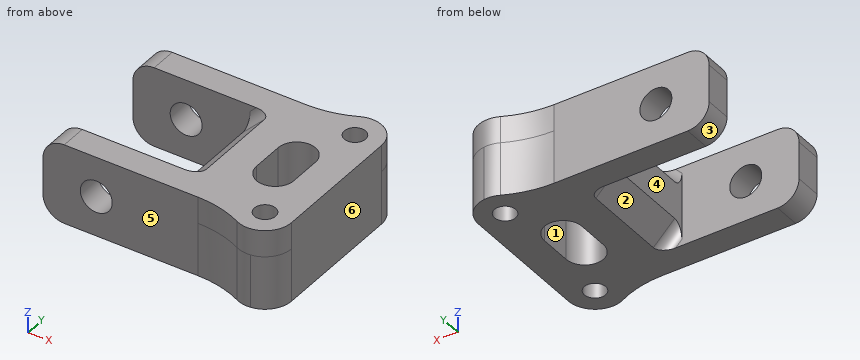
Autodesk Inventor part; units mm, degrees
ref_plane "YZ Plane" through (0, 0, 0) normal (1, 0, 0) x (0, 1, 0)
ref_plane "XZ Plane" through (0, 0, 0) normal (0, 1, 0) x (-1, 0, 0)
ref_plane "XY Plane" through (0, 0, 0) normal (0, 0, 1) x (1, 0, 0)
sketch "Sketch1" plane through (0, 0, 0) normal (0, 0, 1) x (1, 0, 0)
  circle A0 centre (19.8085, -5.5) radius 1
  circle A1 centre (30.8085, -5.5) radius 1
  circle A2 centre (19.8085, 5.5) radius 1
  circle A3 centre (30.8085, 5.5) radius 1
  circle A4 centre (25.3085, 0) radius 6.65
  line L0 (41.3085, 2) -> (41.3085, -2)
  line L1 (35.1065, 2) -> (41.3085, 2)
  arc A5 (35.1065, 2) -> (26.5426, 9.9236) centre (25.3085, 0) ccw
  line L2 (26.5426, 9.9236) -> (-34.0744, 17.4618)
  arc A6 (-34.0744, 17.4618) -> (-39.6915, 12.5) centre (-34.6915, 12.5) ccw
  line L3 (-39.6915, 12.5) -> (-39.6915, -12.5)
  arc A7 (-39.6915, -12.5) -> (-34.0744, -17.4618) centre (-34.6915, -12.5) ccw
  line L4 (-34.0744, -17.4618) -> (26.5426, -9.9236)
  arc A8 (26.5426, -9.9236) -> (35.1065, -2) centre (25.3085, 0) ccw
  line L5 (41.3085, -2) -> (35.1065, -2)
  circle A9 centre (-34.6915, 12.5) radius 2
  circle A10 centre (-34.6915, -12.5) radius 2
  line L6 (-25.1979, 6.2809) -> (9.3489, 1.9847)
  arc A11 (9.3489, -1.9847) -> (9.3489, 1.9847) centre (9.1021, 0) ccw
  line L7 (9.3489, -1.9847) -> (-25.1979, -6.2809)
  arc A12 (-29.6915, -2.3115) -> (-25.1979, -6.2809) centre (-25.6915, -2.3115) ccw
  line L8 (-29.6915, -2.3115) -> (-29.6915, 2.3115)
  arc A13 (-25.1979, 6.2809) -> (-29.6915, 2.3115) centre (-25.6915, 2.3115) ccw
  circle A14 centre (-34.6915, -12.5) radius 5
  circle A15 centre (-34.6915, 12.5) radius 5
  line L9 (-34.6915, -12.5) -> (-34.6915, 12.5)
  line L10 (-34.6915, -12.5) -> (-29.6915, -12.5)
  line L11 (-34.6915, 12.5) -> (-29.6915, 12.5)
  line L12 (-29.6915, 12.5) -> (-29.6915, -12.5)
  line L13 (-34.6915, 0) -> (-64.6915, 0)
  line L14 (-64.6915, -10) -> (-64.6915, 10)
  line L15 (-64.6915, 10) -> (-34.6915, 10)
  line L16 (-34.6915, 10) -> (-34.6915, -10)
  line L17 (-34.6915, -10) -> (-64.6915, -10)
  line L18 (-64.6915, -10) -> (-34.6915, 10) construction
  line L19 (-64.6915, 10) -> (-34.6915, -10) construction
  line L20 (-64.6915, -10) -> (-34.6915, -10)
  line L21 (-34.6915, -10) -> (-34.6915, -15)
  line L22 (-34.6915, -15) -> (-64.6915, -15)
  line L23 (-64.6915, -15) -> (-64.6915, -10)
  line L24 (-64.6915, 10) -> (-34.6915, 10)
  line L25 (-34.6915, 10) -> (-34.6915, 15)
  line L26 (-34.6915, 15) -> (-64.6915, 15)
  line L27 (-64.6915, 15) -> (-64.6915, 10)
  point P0 (0, 0)
  point P1 (-49.6915, 0)
  point P2 (-39.0216, 15)
  point P3 (-39.6915, 10)
  point P4 (-39.6915, -10)
  point P5 (-39.0216, -15)
  dimension "d0" = 10
  dimension "d1" = 10
  dimension "d2" = 30
  dimension "d3" = 20
  dimension "d4" = 30
  dimension "d5" = 30
  dimension "d6" = 5
  dimension "d7" = 30
  dimension "d8" = 5
extrude "Extrusion1" add sketch "Sketch1" along normal blind 10 contours A15 L11 A9 L25 L26 A6 | A7 L22 L21 A10 L10 A14 | L26 L25 A9 L9 L15 A15 A6 | A6 L3 L15 L27 L26 | L12 L8 A14 L9 A15 | A15 L9 A9 L11 | L22 L23 L17 L3 A7 | A7 A14 L17 L9 A10 L21 L22 | L10 A10 L9 A14 | A15 L15 L3 | L9 L13 L3 L15 A15 | A15 L15 L9 | L3 L17 A14 | L9 L17 A14 | A14 L17 L3 L13 L9
thicken "Thicken1" operation add thickness 10 both sides no extend neighbours yes toward (-1, 0, 0) faces at (-64.6915, -11.6667, 3.3333)
thicken "Thicken2" operation add thickness 10 both sides no extend neighbours yes toward (-1, 0, 0) faces at (-64.6915, 13.3333, 3.3333)
sketch "Sketch2" plane through (0, 0, 10) normal (0, 0, 1) x (1, 0, 0)
  line L0 (-39.6915, 10) -> (-39.6915, -10)
  line L1 (-39.6915, -10) -> (-74.6915, -10)
  line L2 (-74.6915, -10) -> (-74.6915, -15)
  line L3 (-74.6915, -15) -> (-39.0216, -15)
  arc A0 (-39.0216, -15) -> (-29.6915, -12.5) centre (-34.6915, -12.5) ccw
  line L4 (-29.6915, -12.5) -> (-29.6915, 12.5)
  arc A1 (-29.6915, 12.5) -> (-39.0216, 15) centre (-34.6915, 12.5) ccw
  line L5 (-39.0216, 15) -> (-74.6915, 15)
  line L6 (-74.6915, 15) -> (-74.6915, 10)
  line L7 (-74.6915, 10) -> (-39.6915, 10)
  circle A2 centre (-34.6915, -12.5) radius 2
  circle A3 centre (-34.6915, 12.5) radius 2
  point P0 (0, 0)
extrude "Extrusion2" add sketch "Sketch2" along normal blind 5
sketch "Sketch3" plane through (0, 0, 15) normal (0, 0, 1) x (1, 0, 0)
  line L0 (-39.6915, 10) -> (-39.6915, -10)
  line L1 (-39.6915, -10) -> (-74.6915, -10)
  line L2 (-74.6915, -10) -> (-74.6915, -15)
  line L3 (-74.6915, -15) -> (-39.0216, -15)
  arc A0 (-39.0216, -15) -> (-29.6915, -12.5) centre (-34.6915, -12.5) ccw
  line L4 (-29.6915, -12.5) -> (-29.6915, 12.5)
  arc A1 (-29.6915, 12.5) -> (-39.0216, 15) centre (-34.6915, 12.5) ccw
  line L5 (-39.0216, 15) -> (-74.6915, 15)
  line L6 (-74.6915, 15) -> (-74.6915, 10)
  line L7 (-74.6915, 10) -> (-39.6915, 10)
  circle A2 centre (-34.6915, -12.5) radius 2
  circle A3 centre (-34.6915, 12.5) radius 2
  line L8 (-39.6915, 10) -> (-39.6915, -10)
  line L9 (-39.6915, 10) -> (-52.6915, 10)
  line L10 (-52.6915, 10) -> (-52.6915, -10)
  line L11 (-52.6915, -10) -> (-39.6915, -10)
  line L12 (-39.6915, -10) -> (-39.6915, 10)
  point P0 (0, 0)
  dimension "d17" = 13
  dimension "d18" = 20
extrude "Extrusion3" add sketch "Sketch3" against normal up to surface (15 mm away) contours L0 L1 L10 L7
chamfer "Chamfer1" distance 4 angle 45 2 edges at (-52.6915, 0, 0) (-52.6915, 0, 15)
fillet "Fillet1" radius 20 2 edges at (-39.0216, -15, 7.5) (-39.0216, 15, 7.5)
sketch "Sketch4" plane through (0, 0, 15) normal (0, 0, 1) x (1, 0, 0)
  line L0 (-48.6915, -10) -> (-74.6915, -10)
  line L1 (-74.6915, -10) -> (-74.6915, -15)
  line L2 (-74.6915, -15) -> (-45.5887, -15)
  arc A0 (-36.8709, -17) -> (-45.5887, -15) centre (-45.5887, -35) ccw
  arc A1 (-36.8709, -17) -> (-29.6915, -12.5) centre (-34.6915, -12.5) ccw
  line L3 (-29.6915, -12.5) -> (-29.6915, 12.5)
  arc A2 (-29.6915, 12.5) -> (-36.8709, 17) centre (-34.6915, 12.5) ccw
  arc A3 (-45.5887, 15) -> (-36.8709, 17) centre (-45.5887, 35) ccw
  line L4 (-45.5887, 15) -> (-74.6915, 15)
  line L5 (-74.6915, 15) -> (-74.6915, 10)
  line L6 (-74.6915, 10) -> (-48.6915, 10)
  line L7 (-48.6915, -10) -> (-48.6915, 10)
  circle A4 centre (-34.6915, -12.5) radius 2
  circle A5 centre (-34.6915, 12.5) radius 2
  circle A6 centre (-34.6915, -12.5) radius 2
  line L8 (-34.6915, 12.5) -> (-34.6915, -12.5)
  line L9 (-34.6915, 0) -> (-39.1915, 0)
  line L10 (-39.1915, 3) -> (-39.1915, -3) construction
  line L11 (-42.6915, 3) -> (-42.6915, -3)
  line L12 (-35.6915, -3) -> (-35.6915, 3)
  arc A7 (-35.6915, 3) -> (-42.6915, 3) centre (-39.1915, 3) ccw
  arc A8 (-42.6915, -3) -> (-35.6915, -3) centre (-39.1915, -3) ccw
  point P0 (0, 0)
  dimension "d25" = 4.5
  dimension "d26" = 3
  dimension "d27" = 7
extrude "Extrusion4" cut sketch "Sketch4" against normal blind 20 contours A7 L12 A8 L11
sketch "Sketch5" plane through (-74.6915, -15, 0) normal (0, -1, 0) x (1, 0, 0)
  line L0 (29.1028, 15) -> (29.1028, 0)
  line L1 (0, 15) -> (29.1028, 15)
  line L2 (0, 0) -> (0, 15)
  line L3 (0, 0) -> (29.1028, 0)
  line L4 (0, 0) -> (0, 15)
  line L5 (0, 7.5) -> (10, 7.5)
  circle A0 centre (10, 7.5) radius 3
  point P0 (74.6915, 0)
  dimension "d30" = 10
  dimension "d31" = 6
extrude "Extrusion5" cut sketch "Sketch5" against normal blind 30 contours A0
fillet "Fillet2" radius 2 4 edges at (-50.6915, 10, 13) (-50.6915, -10, 13) (-50.6915, -10, 2) (-50.6915, 10, 2)
fillet "Fillet3" radius 4 4 edges at (-74.6915, -12.5, 0) (-74.6915, -12.5, 15) (-74.6915, 12.5, 0) (-74.6915, 12.5, 15)
properties part number "2020_fixer_1"
Work out the finished part from the listing and answer in its coordinate system (mm). Face numbers are marked on the shaded views. A direction names the side the tool comes from. Give positions to 0.01 mm unless a question says otherwise; leave off trailing zeros. Loops run counter-clockwise (first coordinate to the right, second up) from the corner with the lowest first, then second, coordinate; pieces in that order, holes last. Notation, with made-up numbers: (37, 26) -> (84, 26) arc R12 ccw to (84, 40) -> close; hole circle Ø9 at (34, 76). An arc over 180 degrees is marked (long way). Use a Markdown table: item, result. Add a question column.
1. Determine the mould class of the marked faces 4, 5 and 6 for opening direction Y: released by +Y, released by -Y, zero draft, split by the parting line, or undercut.
2. Flat-ended cylindrical pins translate along their axes: pin 1 Ø8 at (x, y) = (-69, -8) entering from +Z; pin 2 Ø7.5 at (x, z) = (-65.5, 10.5) entering from -Y; pin 3 Ø3 at (y, z) = (1, 8) entering from -X. Find the tip coordinate at first contact, or state that the pin passes through.
3. For the marked faces 1, 2 and 3, determine the directions among +Z, -Z, +X, -X, +Y, -Y from which every point of the face is accessible in a straight line to the end or side of a thin tool.
4. Find the intervals of material crossed by probe 1 along X at (y, z) = (11.65, 7.5); probe 2 along X at (y, z) = (-12.5, 6); probe 3 along Y at (x, z) = (-54.5, 6.25), in increasing order.
5. Section B-B on x = -60.5 is taken. Determine the outline of the cut face in (y, z).
6. Section C-C on z = 6.25 is taken. Determine the outline of the cut face in (x, y).
7. Section A-A on y = -2 is taken. Determine the outline of the cut face in (x, z), and give its area (3 significant figures).
8. Section D-D on y = -7.5 is taken. Determine the outline of the cut face in (x, z).
Results below:
| question | item | result |
|---|---|---|
| 1 | face 4 | undercut |
| 1 | face 5 | released by -Y |
| 1 | face 6 | zero draft |
| 2 | pin 1 | stops at z = 15 |
| 2 | pin 2 | stops at y = -15 |
| 2 | pin 3 | stops at x = -52.69 |
| 3 | face 1 | +Z, -Z |
| 3 | face 2 | -Z, -X |
| 3 | face 3 | -Z, -X, +Y, -Y |
| 4 | probe 1 | x = -74.69 to -67.69, -61.69 to -36.5, -32.88 to -29.69 |
| 4 | probe 2 | x = -74.69 to -67.29, -62.09 to -36.69, -32.69 to -29.69 |
| 4 | probe 3 | y = -15 to -10, 10 to 15 |
| 5 | outline | (-15, 0) -> (-10, 0) -> (-10, 15) -> (-15, 15) -> close; (10, 0) -> (15, 0) -> (15, 15) -> (10, 15) -> close |
| 6 | outline | (-74.69, -15) -> (-67.42, -15) -> (-67.42, -10) -> (-74.69, -10) -> close; (-74.69, 10) -> (-67.42, 10) -> (-67.42, 15) -> (-74.69, 15) -> close; (-61.96, -15) -> (-45.59, -15) arc R20 cw to (-36.87, -17) arc R5 ccw to (-34.07, -17.46) arc R5 ccw to (-29.69, -12.5) -> (-29.69, 12.5) arc R5 ccw to (-34.07, 17.46) arc R5 ccw to (-36.87, 17) arc R20 cw to (-45.59, 15) -> (-61.96, 15) -> (-61.96, 10) -> (-52.69, 10) -> (-52.69, -10) -> (-61.96, -10) -> close; hole (-42.69, -3) arc R3.5 ccw to (-35.69, -3) -> (-35.69, 3) arc R3.5 ccw to (-42.69, 3) -> close; hole circle Ø4 at (-34.69, -12.5); hole circle Ø4 at (-34.69, 12.5) |
| 7 | outline | (-52.69, 4) -> (-48.69, 0) -> (-42.69, 0) -> (-42.69, 15) -> (-48.69, 15) -> (-52.69, 11) -> close; (-35.69, 0) -> (-29.69, 0) -> (-29.69, 15) -> (-35.69, 15) -> close |
| 7 | area | 224 mm^2 |
| 8 | outline | (-52.69, 4) -> (-48.69, 0) -> (-29.69, 0) -> (-29.69, 15) -> (-48.69, 15) -> (-52.69, 11) -> close |
